CAD build for the part. Positions are in the model's coordinates, mm. A direction names the side the tool comes from. Give positions to 0.01 mm unless a question says otherwise; leave off trailing zeros. Loops run counter-clockwise (first coordinate to the right, second up) from the corner with the lowest first, then second, coordinate; pieces in that order, holes last.
Item 1: Drop flat-ended pins along their axis: P1, Ø1.5, axis at x = 4.5, y = 2, coming from the -Z side; P2, Ø4, axis at x = 18, z = 1, coming from the +Y side; P3, Ø1.5, axis at x = 21, y = -1, coming from the -Z side. Give the stop position or say it passes through.
Item 2: Probe probe 1 along Y at (x, z) = (7.25, 0); probe 2 along Y at (x, z) = (8.5, -2.5); probe 3 along X at (y, z) = (-2.75, 2.5). List the from-to ranges inside material, lowest first.
Item 3: Saw through at A-A on y = 0. Give the cut face in (x, z).
Item 4: Saw through at C-C on x = 10. Give the cut face in (y, z).
Item 5: Which spindle directions (+Z, -Z, +X, -X, +Y, -Y) get a long thin tool onto all of the face, cutting with end or side? Do faces 1 (the flat face through (10, 2.5, 0)), 2 (the flat face through (23.5, 3, 1)), 3 (the flat face through (21.5, -3, -1)), 4 (the flat face through (26, 0, 0)). Say none if no direction does.
Item 6: Saw through at B-B on z = 0. Give the cut face in (x, y).
Item 7: Saw through at D-D on y = 2. Give the cut face in (x, z), plus the area to 3 significant figures.
from build123d import *

# Parameters (mm, degrees)
SKETCH1_R           = 3
BOSS_EXTRUDE1_DEPTH = 26
CUT_EXTRUDE1_DEPTH  = 21.5
SKETCH3_R           = 4
SKETCH3_R_2         = 3
BOSS_EXTRUDE2_DEPTH = 2
BOSS_EXTRUDE3_DEPTH = 1.66


with BuildPart() as part:
    # Sketch1 → Boss-Extrude1 (new body)
    with BuildSketch(Plane(origin=(0, 0, 0), x_dir=(0, 0, -1), z_dir=(1, 0, 0))):
        with Locations(Location((0, 0, 0), (0, 0, 180))):
            Circle(SKETCH1_R)
    extrude(amount=BOSS_EXTRUDE1_DEPTH)

    # Sketch2 → Cut-Extrude1 (cut)
    with BuildSketch(Plane.ZY):
        with BuildLine():
            Line((-1.658312395, 2.5), (1.658312395, 2.5))
            ThreePointArc((1.658312395, 2.5), (0, 3), (-1.658312395, 2.5))
        make_face()
    extrude(amount=-CUT_EXTRUDE1_DEPTH, mode=Mode.SUBTRACT)

    # Sketch3 → Boss-Extrude2 (add)
    with BuildSketch(Plane.ZY.offset(-21.5)):
        Circle(SKETCH3_R)
        Circle(SKETCH3_R_2, mode=Mode.SUBTRACT)
    extrude(amount=-BOSS_EXTRUDE2_DEPTH)

    # Sketch4 → Boss-Extrude3 (add, symmetric)
    with BuildSketch(Plane.XY):
        Polygon((21, 2.5), (21.5, 2.75), (21.5, 2.5), align=None)
    extrude(amount=BOSS_EXTRUDE3_DEPTH, both=True)


solid = part.part
Results below:
1. P1: stops at z = -2.73
1. P2: stops at y = 2.5
1. P3: stops at z = -3.98
2. probe 1: y = -3 to 2.5
2. probe 2: y = -1.66 to 1.66
2. probe 3: x = 21.5 to 23.5
3. outline: (0, -3) - (21.5, -3) - (21.5, -4) - (23.5, -4) - (23.5, -3) - (26, -3) - (26, 3) - (23.5, 3) - (23.5, 4) - (21.5, 4) - (21.5, 3) - (0, 3) - close
4. outline: (2.5, -1.66) - (2.5, 1.66) arc R3 ccw (long way) to start
5. face 1: +Z, -Z, -X, +Y
5. face 2: +X
5. face 3: -X
5. face 4: +Z, -Z, +X, +Y, -Y
6. outline: (0, -3) - (21.5, -3) - (21.5, -4) - (23.5, -4) - (23.5, -3) - (26, -3) - (26, 3) - (23.5, 3) - (23.5, 4) - (21.5, 4) - (21.5, 2.75) - (21, 2.5) - (0, 2.5) - close
7. outline: (0, -2.24) - (21.5, -2.24) - (21.5, -3.46) - (23.5, -3.46) - (23.5, -2.24) - (26, -2.24) - (26, 2.24) - (23.5, 2.24) - (23.5, 3.46) - (21.5, 3.46) - (21.5, 2.24) - (0, 2.24) - close
7. area: 121 mm2
